Geometry: final body of the model. Coordinates: model frame, mm. Give positions to 0.01 mm unless a question says otherwise; leave off trailing zeros. Write each loop counter-clockwise with the first axis right and the second up, starting at its lowest first coordinate (ties: lowest second). Pieces come first, ordered by that corner, then holes. Notation, with made-up numbers: (-27.5, 62) -> (28.5, 62) arc R25 ccw to (28.5, 91) -> close; hole circle Ø2 at (8.25, 14). An arc over 180 degrees is marked (long way). Answer as a JSON object with one key per item and string values. Group by question number.
(1) Contact query for a flat-ended pin moving along its axis: pin 1 Ø4 at (x, y) = (60, -1) entering from -Z. Output: stop coordinate, or through.
(2) Section query D-D on z = 1.5. State how many separate pieces and enclosed holes the cut face has, plus the area to 3 significant figures.
(3) Section query C-C on x = -20.5. Output: boundary loops of the cut face in (y, z), plus the area to 3 significant figures.
(4) Section query B-B on x = -62.5. Output: boundary loops of the cut face in (y, z), plus the area to 3 significant figures.
(5) Material intervals for probe 1 along X at (y, z) = (-50.5, 1.7); probe 2 along Y at (x, z) = (0, 1.8); probe 3 along X at (y, z) = (-29.5, 1.35), sorted ascending.
(6) Section query A-A on y = -100. Output: boundary loops of the cut face in (x, z), plus the area to 3 significant figures.
from build123d import *

# Parameters (mm, degrees)
SKETCH_W        = 155
SKETCH_H        = 160
PAD_DEPTH       = 2.5
SKETCH001_W     = 15.25
SKETCH001_H     = 10.25
POCKET_DEPTH    = 2.5
SKETCH002_R     = 2.625
POCKET001_DEPTH = 2.5


with BuildPart() as part:
    # Sketch → Pad (new body)
    with BuildSketch(Plane.XY):
        with Locations((0.10674, -30.909095)):
            Rectangle(SKETCH_W, SKETCH_H)
    extrude(amount=PAD_DEPTH)

    # Sketch001 (on Face6 of Pad) → Pocket (cut)
    with BuildSketch(Plane.XY.offset(2.5)):
        with Locations((-64.76826, 38.965905)):
            Rectangle(SKETCH001_W, SKETCH001_H)
        with Locations((-64.76826, -100.784095)):
            Rectangle(SKETCH001_W, SKETCH001_H)
    extrude(amount=-POCKET_DEPTH, mode=Mode.SUBTRACT)

    # Sketch002 (on Face5 of Pocket) → Pocket001 (cut)
    with BuildSketch(Plane.XY.offset(2.5)):
        with Locations((-19.89326, -30.909095)):
            Circle(SKETCH002_R)
        with Locations((-39.89326, -30.909095)):
            Circle(SKETCH002_R)
        with Locations((0.10674, -30.909095)):
            Circle(SKETCH002_R)
        with Locations((20.10674, -30.909095)):
            Circle(SKETCH002_R)
        with Locations((40.10674, -30.909095)):
            Circle(SKETCH002_R)
        with Locations((-39.89326, -10.909095)):
            Circle(SKETCH002_R)
        with Locations((-19.89326, -10.909095)):
            Circle(SKETCH002_R)
        with Locations((0.10674, -10.909095)):
            Circle(SKETCH002_R)
        with Locations((20.10674, -10.909095)):
            Circle(SKETCH002_R)
        with Locations((40.10674, -10.909095)):
            Circle(SKETCH002_R)
        with Locations((-39.89326, -50.909095)):
            Circle(SKETCH002_R)
        with Locations((-19.89326, -50.909095)):
            Circle(SKETCH002_R)
        with Locations((0.10674, -50.909095)):
            Circle(SKETCH002_R)
        with Locations((20.10674, -50.909095)):
            Circle(SKETCH002_R)
        with Locations((40.10674, -50.909095)):
            Circle(SKETCH002_R)
        with Locations((-39.89326, -70.909095)):
            Circle(SKETCH002_R)
        with Locations((-19.89326, -70.909095)):
            Circle(SKETCH002_R)
        with Locations((0.10674, -70.909095)):
            Circle(SKETCH002_R)
        with Locations((20.10674, -70.909095)):
            Circle(SKETCH002_R)
        with Locations((40.10674, -70.909095)):
            Circle(SKETCH002_R)
        with Locations((-39.89326, 9.090905)):
            Circle(SKETCH002_R)
        with Locations((-19.89326, 9.090905)):
            Circle(SKETCH002_R)
        with Locations((0.10674, 9.090905)):
            Circle(SKETCH002_R)
        with Locations((20.10674, 9.090905)):
            Circle(SKETCH002_R)
        with Locations((40.10674, 9.090905)):
            Circle(SKETCH002_R)
    extrude(amount=-POCKET001_DEPTH, mode=Mode.SUBTRACT)


solid = part.part
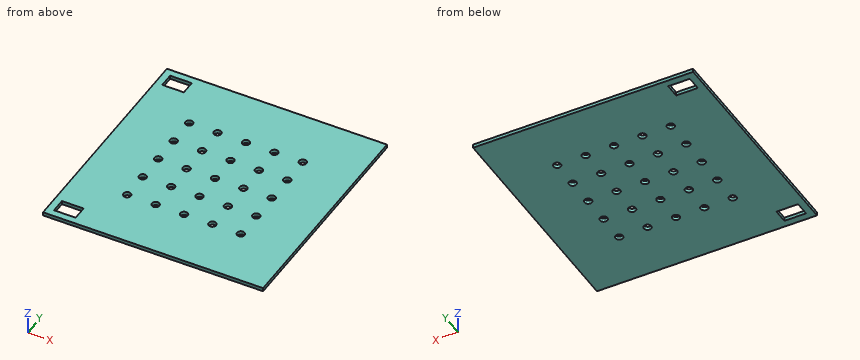
Answer list:
{
 "1": {"pin 1": "z = 0"},
 "2": {"separate pieces": "1", "enclosed holes": "27", "area": "23,900 mm2"},
 "3": {"outline": "(-110.91, 0) -> (-73.46, 0) -> (-73.46, 2.5) -> (-110.91, 2.5) -> close; (-68.36, 0) -> (-53.46, 0) -> (-53.46, 2.5) -> (-68.36, 2.5) -> close; (-48.36, 0) -> (-33.46, 0) -> (-33.46, 2.5) -> (-48.36, 2.5) -> close; (-28.36, 0) -> (-13.46, 0) -> (-13.46, 2.5) -> (-28.36, 2.5) -> close; (-8.36, 0) -> (6.54, 0) -> (6.54, 2.5) -> (-8.36, 2.5) -> close; (11.64, 0) -> (49.09, 0) -> (49.09, 2.5) -> (11.64, 2.5) -> close", "area": "336 mm2"},
 "4": {"outline": "(-110.91, 0) -> (-105.91, 0) -> (-105.91, 2.5) -> (-110.91, 2.5) -> close; (-95.66, 0) -> (33.84, 0) -> (33.84, 2.5) -> (-95.66, 2.5) -> close; (44.09, 0) -> (49.09, 0) -> (49.09, 2.5) -> (44.09, 2.5) -> close", "area": "349 mm2"},
 "5": {"probe 1": "-77.39 to -42.49, -37.3 to -22.49, -17.3 to -2.49, 2.7 to 17.51, 22.7 to 37.51, 42.7 to 77.61", "probe 2": "-110.91 to -73.53, -68.29 to -53.53, -48.29 to -33.53, -28.29 to -13.53, -8.29 to 6.47, 11.71 to 49.09", "probe 3": "-77.39 to -42.11, -37.68 to -22.11, -17.68 to -2.11, 2.32 to 17.89, 22.32 to 37.89, 42.32 to 77.61"},
 "6": {"outline": "(-77.39, 0) -> (-72.39, 0) -> (-72.39, 2.5) -> (-77.39, 2.5) -> close; (-57.14, 0) -> (77.61, 0) -> (77.61, 2.5) -> (-57.14, 2.5) -> close", "area": "349 mm2"}
}
